from build123d import *

# Parameters (mm, degrees)
SKETCH2_W           = 36
SKETCH2_H           = 42
BOSS_EXTRUDE1_DEPTH = 12
CUT_EXTRUDE1_DEPTH  = 15
CUT_EXTRUDE2_DEPTH  = 12
SKETCH5_W           = 30
SKETCH5_H           = 1.695405108
CUT_EXTRUDE3_DEPTH  = 25
SKETCH6_R           = 4.25
CUT_EXTRUDE4_DEPTH  = 7.1
SKETCH7_W           = 2
SKETCH7_H           = 12
BOSS_EXTRUDE2_DEPTH = 42


with BuildPart() as part:
    # Sketch2 → Boss-Extrude1 (new body)
    with BuildSketch(Plane.XY):
        with Locations((-1.487179487, 11.461538462)):
            Rectangle(SKETCH2_W, SKETCH2_H)
    extrude(amount=BOSS_EXTRUDE1_DEPTH)

    # Sketch3 → Cut-Extrude1 (cut)
    with BuildSketch(Plane(origin=(0, 32.461538462, 0), x_dir=(1, 0, 0), z_dir=(0, 1, 0))):
        Polygon((-18.087179487, -12), (-18.736956279, -9.575), (-15.212402696, -9.575), (-15.862179487, -12), align=None)
        Polygon((15.112820513, -12), (15.762597304, -9.575), (12.238043721, -9.575), (12.887820513, -12), align=None)
    extrude(amount=-CUT_EXTRUDE1_DEPTH, mode=Mode.SUBTRACT)

    # Sketch4 → Cut-Extrude2 (cut)
    with BuildSketch(Plane.XY.offset(12)):
        with BuildLine():
            Line((-10.823469947, 32.461538462), (7.849110972, 32.461538462))
            Line((7.849110972, 32.461538462), (7.849110972, 21.461538462))
            ThreePointArc((7.849110972, 21.461538462), (-1.487179487, 12.125248002), (-10.823469947, 21.461538462))
            Line((-10.823469947, 21.461538462), (-10.823469947, 32.461538462))
        make_face()
    extrude(amount=-CUT_EXTRUDE2_DEPTH, mode=Mode.SUBTRACT)

    # Sketch5 → Cut-Extrude3 (cut)
    with BuildSketch(Plane(origin=(0, 32.461538462, 0), x_dir=(1, 0, 0), z_dir=(0, 1, 0))):
        with Locations((-1.487179487, -6)):
            Rectangle(SKETCH5_W, SKETCH5_H)
    extrude(amount=-CUT_EXTRUDE3_DEPTH, mode=Mode.SUBTRACT)

    # Sketch6 → Cut-Extrude4 (cut)
    with BuildSketch(Plane.XY.offset(12)):
        with Locations((-1.509360089, 6.461538462)):
            Circle(SKETCH6_R)
    extrude(amount=-CUT_EXTRUDE4_DEPTH, mode=Mode.SUBTRACT)

    # Sketch7 → Boss-Extrude2 (add)
    with BuildSketch(Plane(origin=(0, 32.461538462, 0), x_dir=(1, 0, 0), z_dir=(0, 1, 0))):
        with Locations((-20.487179487, -6)):
            Rectangle(SKETCH7_W, SKETCH7_H)
        with Locations((17.512820513, -6)):
            Rectangle(SKETCH7_W, SKETCH7_H)
    extrude(amount=-BOSS_EXTRUDE2_DEPTH)


solid = part.part
Geometry: final body of the model. Coordinates: model frame, mm. A direction names the side the tool comes from. Give positions to 0.01 mm unless a question says otherwise; leave off trailing zeros. Order: outer loops, then holes, each group sorted by start corner. A loop starts at its lowest first (then second) coordinate and runs counter-clockwise, first axis right, second up. Notation, with made-up numbers: (76.5, 61.5) -> (96.5, 61.5) arc R18 cw to (96.5, 65.5) -> close; hole circle Ø9 at (-34, -29.5). An arc over 180 degrees is marked (long way). Answer as a JSON object with one key per item and string values.
Q1. Section C-C (z = 6.25). Output: boundary loops of the cut face in (x, y), plus the area to 3 significant figures.
Entries:
{"outline": "(-21.49, -9.54) -> (18.51, -9.54) -> (18.51, 32.46) -> (13.51, 32.46) -> (13.51, 7.46) -> (2.62, 7.46) arc R4.25 cw (long way) to (-5.64, 7.46) -> (-16.49, 7.46) -> (-16.49, 32.46) -> (-21.49, 32.46) -> close", "area": "893 mm^2"}
Q2. Section A-A (y = 29.5). Output: boundary loops of the cut face in (x, z) (3 decimals), plus the area to 3 significant figures.
Entries:
{"outline": "(-21.487, 0) -> (-10.823, 0) -> (-10.823, 5.152) -> (-16.487, 5.152) -> (-16.487, 6.848) -> (-10.823, 6.848) -> (-10.823, 12) -> (-15.862, 12) -> (-15.212, 9.575) -> (-18.737, 9.575) -> (-18.087, 12) -> (-21.487, 12) -> close; (7.849, 0) -> (18.513, 0) -> (18.513, 12) -> (15.113, 12) -> (15.763, 9.575) -> (12.238, 9.575) -> (12.888, 12) -> (7.849, 12) -> (7.849, 6.848) -> (13.513, 6.848) -> (13.513, 5.152) -> (7.849, 5.152) -> close", "area": "223 mm^2"}
Q3. Section D-D (x = -6.5). Output: boundary loops of the cut face in (y, z).
Entries:
{"outline": "(-9.54, 0) -> (13.59, 0) -> (13.59, 5.15) -> (7.46, 5.15) -> (7.46, 6.85) -> (13.59, 6.85) -> (13.59, 12) -> (-9.54, 12) -> close"}
Q4. Section B-B (x = -0.5). Output: boundary loops of the cut face in (y, z).
Entries:
{"outline": "(-9.54, 0) -> (12.18, 0) -> (12.18, 5.15) -> (10.59, 5.15) -> (10.59, 4.9) -> (2.33, 4.9) -> (2.33, 12) -> (-9.54, 12) -> close; (10.59, 6.85) -> (12.18, 6.85) -> (12.18, 12) -> (10.59, 12) -> close"}
Q5. First-contact query: pin 1 (0.5 mm diameter, centred on x = -12, z = 6.5, fed in from +Y); pin 2 (1.8 mm diameter, centred on x = -17, y = 22, fed in from +Z) (3 decimals); pin 3 (2.5 mm diameter, centred on x = -0.5, y = 7.5, fed in from +Z); pin 4 (11 mm diameter, centred on x = -1.51, y = 6.46, fed in from +Z). Flat tips, straight axial feed; report the tip coordinate or a pass-through.
Entries:
{"pin 1": "stops at y = 7.46", "pin 2": "stops at z = 9.575", "pin 3": "stops at z = 4.9", "pin 4": "stops at z = 12"}
Q6. Access query for faces 4 (the flat face through (-18.41, 25.07, 10.8)), 5 (the flat face through (7.849, 27, 3)), 6 (the cylindrical face through (-2.431, 2.313, 8.5)), 7 (the flat face through (-2, -9.538, 6)). Directions: +Z, -Z, +X, -X, +Y, -Y. A direction counts if a zero-diameter tool reaches every point of the face in a straight line with its end or side. Return the directions, or none.
Entries:
{"face 4": "+Y", "face 5": "+Z, -Z, +Y", "face 6": "+Z", "face 7": "+Z, -Z, +X, -X, -Y"}
Q7. Draft query along Z for faces 1 (the flat face through (8, 7.462, 6)), 2 (the flat face through (-2, 7, 4.9)), 3 (the flat face through (-16, 32.462, 5)). Return one class per face: released by +Z, released by -Z, zero draft, split by the parting line, or undercut.
Entries:
{"face 1": "undercut", "face 2": "released by +Z", "face 3": "zero draft"}
Q8. Material intervals for probe 1 along Z at (x, y) = (-11, 14.5); probe 2 along X at (y, z) = (29, 10.5); probe 3 along X at (y, z) = (27.5, 0.75), sorted ascending.
Entries:
{"probe 1": "z = 0 to 5.15, 6.85 to 12", "probe 2": "x = -21.49 to -18.49, -15.46 to -10.82, 7.85 to 12.49, 15.51 to 18.51", "probe 3": "x = -21.49 to -10.82, 7.85 to 18.51"}
